```python
from build123d import *

# Parameters (mm, degrees)
SZKIC1_W                    = 46
SZKIC1_H                    = 21
DODANIE_WYCI_GNI_CIE1_DEPTH = 10
SZKIC2_R                    = 8
DODANIE_WYCI_GNI_CIE2_DEPTH = 11
DODANIE_WYCI_GNI_CIE3_DEPTH = 4
SZKIC4_R                    = 0.6
DODANIE_WYCI_GNI_CIE4_DEPTH = 1.5
SFAZOWANIE1_SIZE            = 0.5


with BuildPart() as part:
    # Szkic1 → Dodanie-wyciągnięcie1 (new body)
    with BuildSketch(Plane.XY):
        Rectangle(SZKIC1_W, SZKIC1_H)
    extrude(amount=DODANIE_WYCI_GNI_CIE1_DEPTH)

    # Szkic2 → Dodanie-wyciągnięcie2 (add)
    with BuildSketch(Plane.XY.offset(10)):
        with Locations(Location((-13, 0, 0), (0, 0, 180))):
            Circle(SZKIC2_R)
        with Locations(Location((13, 0, 0), (0, 0, 180))):
            Circle(SZKIC2_R)
    extrude(amount=DODANIE_WYCI_GNI_CIE2_DEPTH)

    # Szkic3 → Dodanie-wyciągnięcie3 (add)
    with BuildSketch(Plane.XY.offset(10)):
        with BuildLine():
            Line((-3, -5.5), (3, -5.5))
            ThreePointArc((3, -5.5), (5, -7.5), (3, -9.5))
            Line((3, -9.5), (-3, -9.5))
            ThreePointArc((-3, -9.5), (-5, -7.5), (-3, -5.5))
        make_face()
    extrude(amount=DODANIE_WYCI_GNI_CIE3_DEPTH)

    # Szkic4 → Dodanie-wyciągnięcie4 (add)
    with BuildSketch(Plane.XY.offset(10)):
        with Locations(Location((-3.66, 9.3, 0), (0, 0, 180))):
            Circle(SZKIC4_R)
        with Locations(Location((-1.22, 9.3, 0), (0, 0, 180))):
            Circle(SZKIC4_R)
        with Locations(Location((3.66, 9.3, 0), (0, 0, 180))):
            Circle(SZKIC4_R)
        with Locations(Location((1.22, 9.3, 0), (0, 0, 180))):
            Circle(SZKIC4_R)
    extrude(amount=DODANIE_WYCI_GNI_CIE4_DEPTH)

    # Sfazowanie1
    sfazowanie1_edges = [part.edges().sort_by_distance(p)[0] for p in [
        (-3.06, 9.3, 11.5),
        (-0.62, 9.3, 11.5),
        (4.26, 9.3, 11.5),
        (1.82, 9.3, 11.5),
    ]]
    chamfer(sfazowanie1_edges, length=SFAZOWANIE1_SIZE)


solid = part.part
```
Geometry check sheet. Reference: the model listing, model coordinates, mm. A direction names the side the tool comes from. Round coordinates to 2 decimals unless told otherwise and drop trailing zeros. Write each loop counter-clockwise with the first axis right and the second up, starting at its lowest first coordinate (ties: lowest second). Pieces come first, ordered by that corner, then holes. Notation, with made-up numbers: (71.5, -20) -> (118.5, -20) arc R23 cw to (118.5, 6) -> close; hole circle Ø3 at (47.25, -2.5). An arc over 180 degrees is marked (long way). Put each result on its own line as item: value.
1) Cross-section at A-A, the plane z = 13. Enter the section's corners in (x, y), plus the area to 3 significant figures.
Recorded:
outline: circle Ø16 at (-13, 0); (-3, -9.5) -> (3, -9.5) arc R2 ccw to (3, -5.5) -> (-3, -5.5) arc R2 ccw to start; circle Ø16 at (13, 0)
area: 439 mm2
2) Access from +Z, -Z, +X, -X, +Y, -Y to the whole of each face (thin tool, end or side, straight path). Record for faces 4 (the face through (14.73, 7.81, 15.42)), 5 (the face through (0, 10.5, 5)).
Recorded:
face 4: +Z
face 5: +Z, -Z, +X, -X, +Y
3) Thickness scan on probe 1 along Y at (x, z) = (13, 16.75); probe 2 along Z at (x, y) = (0, 9.25); probe 3 along X at (y, z) = (4.5, 11.5). Record the ranges inside material, lowest first. Write a range as from..to.
Recorded:
probe 1: y = -8..8
probe 2: z = 0..10
probe 3: x = -19.61..-6.39, 6.39..19.61
4) Cross-section at D-D, the plane y = -3.75. Enter the section's corners in (x, z), plus the area to 3 significant figures.
Recorded:
outline: (-23, 0) -> (23, 0) -> (23, 10) -> (20.07, 10) -> (20.07, 21) -> (5.93, 21) -> (5.93, 10) -> (-5.93, 10) -> (-5.93, 21) -> (-20.07, 21) -> (-20.07, 10) -> (-23, 10) -> close
area: 771 mm2
5) Cross-section at C-C, the plane y = 2. Enter the section's corners in (x, z), plus the area to 3 significant figures.
Recorded:
outline: (-23, 0) -> (23, 0) -> (23, 10) -> (20.75, 10) -> (20.75, 21) -> (5.25, 21) -> (5.25, 10) -> (-5.25, 10) -> (-5.25, 21) -> (-20.75, 21) -> (-20.75, 10) -> (-23, 10) -> close
area: 801 mm2
6) Release check for a two-part mould opening along Y. For faces 1 (the face through (0, -9.5, 12)), 2 (the face through (5, -7.5, 12)), 3 (the face through (23, 0, 5)) record: pulls with the +Y half, pulls with the -Y half, needs draft (parallel to the pull), parting line crosses it, or undercut.
Recorded:
face 1: pulls with the -Y half
face 2: undercut
face 3: needs draft
7) Cross-section at B-B, the plane x = -13. Enter the section's corners in (y, z).
Recorded:
outline: (-10.5, 0) -> (10.5, 0) -> (10.5, 10) -> (8, 10) -> (8, 21) -> (-8, 21) -> (-8, 10) -> (-10.5, 10) -> close
8) Depth check by flat-ended pin: P1, Ø3, axis at x = 0.5, y = -8.5, coming from the +Z side; P2, Ø8, axis at y = -2, z = 15.5, coming from the +X side; P3, Ø4.5, axis at x = -1, z = 11.5, coming from the +Y side; P4, Ø3, axis at x = 18, z = 13, coming from the +Y side. Enter the tip coordinate at first touch or a pass-through.
Recorded:
P1: stops at z = 14
P2: stops at x = 21
P3: stops at y = 10.5
P4: stops at y = 7.19
